Source: CAD feature listing. Evaluate the final solid. Frame: model axes, mm. Give positions to 0.01 mm unless a question says otherwise; leave off trailing zeros. Loops run counter-clockwise (first coordinate to the right, second up) from the corner with the lowest first, then second, coordinate; pieces in that order, holes last.
```python
from build123d import *

# Parameters (mm, degrees)
KES_EKSTR_ZYON1_DEPTH      = 139.907343218
KES_EKSTR_ZYON1_DEPTH_BACK = 19
IZIM11_R                   = 6.5


with BuildPart() as part:
    # izim4 → D_nd_r2 (revolve)
    with BuildSketch(Plane.XY):
        with BuildLine():
            Line((17.5, 0), (-17.5, 0))
            ThreePointArc((-17.5, 0), (0, 17.5), (17.5, 0))
        make_face()
    revolve(axis=Axis((-17.5, 0, 0), (1, 0, 0)))



with BuildPart() as body_2:
    # izim6 → D_nd_r3 (revolve)
    with BuildSketch(Plane.XY, mode=Mode.PRIVATE) as d_nd_r3_sk:
        with BuildLine():
            Line((34.395313644, 10.5), (53.604686356, 10.5))
            ThreePointArc((53.604686356, 10.5), (54.665346528, 10.263846285), (55.525623627, 9.6))
            ThreePointArc((55.525623627, 9.6), (58.104686356, 5.104686356), (59, 0))
            Line((59, 0), (29, 0))
            ThreePointArc((29, 0), (29.895313644, 5.104686356), (32.474376373, 9.6))
            ThreePointArc((32.474376373, 9.6), (33.334653472, 10.263846285), (34.395313644, 10.5))
        make_face()
    revolve(d_nd_r3_sk.sketch.rotate(Axis((59, 0, 0), (-1, 0, 0)), 90), axis=Axis((59, 0, 0), (-1, 0, 0)))


with BuildPart() as body_3:
    # izim7 → D_nd_r4 (revolve)
    with BuildSketch(Plane.XY):
        with BuildLine():
            Line((86, 0), (110, 0))
            ThreePointArc((110, 0), (98, 12), (86, 0))
        make_face()
    revolve(axis=Axis((86, 0, 0), (1, 0, 0)))


with BuildPart() as part_1:
    add(part.part)

    add(body_2.part)  # D_nd_r5 merges body 2

    add(body_3.part)  # D_nd_r5 merges body 3
    # izim8 → D_nd_r5 (revolve)
    with BuildSketch(Plane.XY, mode=Mode.PRIVATE) as d_nd_r5_sk:
        with BuildLine():
            Line((15.00833102, 9), (87.334635496, 5.5))
            ThreePointArc((87.334635496, 5.5), (86.338431194, 2.82980794), (86, 0))
            Line((86, 0), (17.5, 0))
            ThreePointArc((17.5, 0), (16.865583193, 4.669272275), (15.00833102, 9))
        make_face()
    revolve(d_nd_r5_sk.sketch.rotate(Axis((86, 0, 0), (-1, 0, 0)), 180), axis=Axis((86, 0, 0), (-1, 0, 0)))

    # izim10 → D_nd_r6 (revolve)
    with BuildSketch(Plane.XY, mode=Mode.PRIVATE) as d_nd_r6_sk:
        with BuildLine():
            Line((98, 83), (98, 9.392026888))
            ThreePointArc((98, 9.392026888), (91.636038969, 12.028065858), (89, 18.392026888))
            ThreePointArc((89, 18.392026888), (92.993500576, 32.475023678), (89.599731438, 46.714446998))
            ThreePointArc((89.599731438, 46.714446998), (86.708723874, 65.750824244), (96.377409163, 82.401893523))
            ThreePointArc((96.377409163, 82.401893523), (97.135342209, 82.845712451), (98, 83))
        make_face()
    revolve(d_nd_r6_sk.sketch.rotate(Axis((98, 83, 0), (0, -1, 0)), 270), axis=Axis((98, 83, 0), (0, -1, 0)))

    # izim11 → Kes-Ekstr_zyon1 (cut, two sides: drawn at the far end of the back side and taken through both)
    with BuildSketch(Plane(origin=(0, 0, 0), x_dir=(1, 0, 0), z_dir=(0, 1, 0)).offset(-KES_EKSTR_ZYON1_DEPTH_BACK)):
        with Locations(Location((44, 0, 0), (0, 0, 90))):
            Circle(IZIM11_R)
    extrude(amount=KES_EKSTR_ZYON1_DEPTH + KES_EKSTR_ZYON1_DEPTH_BACK, mode=Mode.SUBTRACT)


solid = part_1.part
```
(1) Section C-C, the plane y = 23. Return the cut outline in (x, z).
A:
outline: circle Ø13.62 at (98, 0)
(2) First-contact query: pin 1 (6 mm diameter, centred on x = 92, z = -2, fed in from +Y); pin 2 (8 mm diameter, centred on x = 92, z = 8.5, fed in from +Y); pin 3 (6 mm diameter, centred on y = 67, z = 4.5, fed in from +X). Flat tips, straight axial feed; report the tip coordinate or a pass-through.
A:
pin 1: stops at y = 80.83
pin 2: stops at y = 77.19
pin 3: stops at x = 109.2
(3) Section A-A, the plane x = 44. Return the cut outline in (y, z).
A:
outline: (-8.25, -6.5) arc R10.5 ccw to (8.25, -6.5) - close; (-8.25, 6.5) - (8.25, 6.5) arc R10.5 ccw to start
(4) Mould query, pull axis Z, two halves, no side actions, for faces 1 (the cylindrical face through (38.519, -0.147, -3.494)), 2 (the conical face through (72.52, -5.93, 1.87)). Classes: pulls with the +Z half, pulls with the -Z half, needs draft (parallel to the pull), parting line crosses it, or undercut.
A:
face 1: undercut
face 2: parting line crosses it
(5) Section B-B, the plane x = 5. Return the cut outline in (y, z), then the cut area to 3 significant figures.
A:
outline: circle Ø33.54 at (0, 0)
area: 884 mm2
(6) Ray query, line 1 along Y through (x, z) = (104, -4); line 2 along X through (y, z) = (-4.5, 0); line 3 along X through (y, z) = (1, 0). Return the intervals inside material, ascending.
A:
line 1: y = -9.59 to 9.59, 13.01 to 21.98, 44.2 to 76
line 2: x = -16.91 to 37.5, 50.5 to 109.12
line 3: x = -17.47 to 37.5, 50.5 to 109.96
